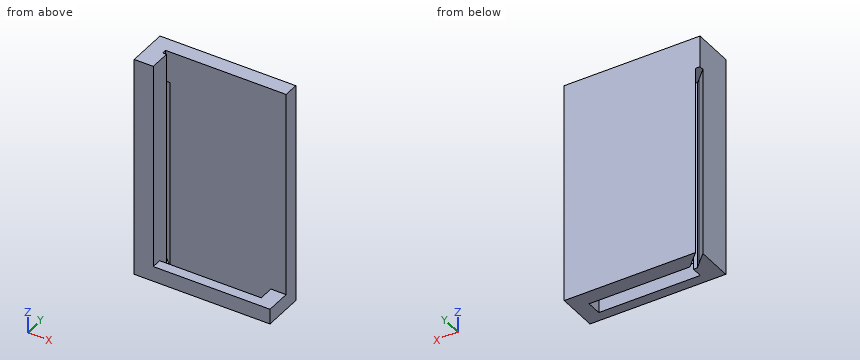
from build123d import *

# Parameters (mm, degrees)
F1_DEPTH = 25
F2_DEPTH = 150
F4_DEPTH = 175
F5_W     = 12
F5_H     = 8
F5_H_2   = 12
F6_DEPTH = 12


with BuildPart() as f1:
    # F0 (on Top) → F1 (new body)
    with BuildSketch(Plane.XY):
        Polygon((-15.4107665035, -11.7272357842), (-11.8752325976, -15.2627696901), (79.5892334965, -15.2627696901), (79.5892334965, -3.2627696901), (-15.4107665035, -3.2627696901), align=None)
        Polygon((-23.8752325976, -3.2627696901), (-15.4107665035, -11.7272357842), (-15.4107665035, -3.2627696901), align=None)
        Polygon((-18.9463004094, -15.2627696901), (-15.4107665035, -15.2627696901), (-27.4107665035, -3.2627696901), (-27.4107665035, -6.7983035961), align=None)
        Polygon((-27.4107665035, -15.2627696901), (-18.9463004094, -15.2627696901), (-27.4107665035, -6.7983035961), align=None)
        Polygon((-15.4107665035, -18.7983035961), (-18.9463004094, -15.2627696901), (-27.4107665035, -15.2627696901), (-27.4107665035, -35.2627696901), (-15.4107665035, -35.2627696901), align=None)
        Polygon((-27.4107665035, -3.2627696901), (-15.4107665035, -15.2627696901), (-15.4107665035, -11.7272357842), (-23.8752325976, -3.2627696901), align=None)
        Polygon((-15.4107665035, -11.7272357842), (-15.4107665035, -15.2627696901), (-11.8752325976, -15.2627696901), align=None)
        Polygon((-15.4107665035, -18.7983035961), (-15.4107665035, -15.2627696901), (-18.9463004094, -15.2627696901), align=None)
    extrude(amount=F1_DEPTH)

    # F0 (on Top) → F2 (join)
    with BuildSketch(Plane.XY):
        Polygon((-15.4107665035, -18.7983035961), (-18.9463004094, -15.2627696901), (-27.4107665035, -15.2627696901), (-27.4107665035, -35.2627696901), (-15.4107665035, -35.2627696901), align=None)
        Polygon((-23.8752325976, -3.2627696901), (-15.4107665035, -11.7272357842), (-15.4107665035, -3.2627696901), align=None)
        Polygon((-15.4107665035, -11.7272357842), (-11.8752325976, -15.2627696901), (79.5892334965, -15.2627696901), (79.5892334965, -3.2627696901), (-15.4107665035, -3.2627696901), align=None)
        Polygon((-27.4107665035, -15.2627696901), (-18.9463004094, -15.2627696901), (-27.4107665035, -6.7983035961), align=None)
    extrude(amount=-F2_DEPTH)

    # F3 (on face) → F4 (join, through all)
    with BuildSketch(Plane(origin=(0, 0, -150), x_dir=(1, 0, 0), z_dir=(0, 0, -1))):
        Polygon((-15.4107665035, 30.7983035961), (-15.4107665035, 18.7983035961), (-12.4107665035, 18.7983035961), (-12.4107665035, 30.7983035961), (-12.4107665035, 35.2627696901), (-15.4107665035, 35.2627696901), align=None)
    extrude(amount=-F4_DEPTH)

    # F5 (on face) → F6 (join)
    with BuildSketch(Plane(origin=(0, 0, -150), x_dir=(1, 0, 0), z_dir=(0, 0, -1))):
        Polygon((-12.4107665035, 35.2627696901), (-12.4107665035, 30.7983035961), (-12.4107665035, 27.2627696901), (67.5892334965, 27.2627696901), (67.5892334965, 35.2627696901), align=None)
        with Locations((73.5892334965, 31.2627696901)):
            Rectangle(F5_W, F5_H)
        with Locations((73.5892334965, 21.2627696901)):
            Rectangle(F5_W, F5_H_2)
        Polygon((79.5892334965, 15.2627696901), (67.5892334965, 15.2627696901), (-11.8752325976, 15.2627696901), (-23.8752325976, 3.2627696901), (79.5892334965, 3.2627696901), align=None)
    extrude(amount=-F6_DEPTH)


solid = f1.part
Geometry: final body of the model. Coordinates: model frame, mm. Round coordinates to 2 decimals unless told otherwise and drop trailing zeros. Loops run counter-clockwise (first coordinate to the right, second up) from the corner with the lowest first, then second, coordinate; pieces in that order, holes last.
Q1. Material intervals for L1, parallel to Z at x = 50, y = -31; L2, parallel to Y at x = 37, z = -90.5; L3, parallel to X at y = -7, z = -120.5, sorted ascending.
Q2. Pin query (flat end, axial travel): P1, Ø3, axis at y = -23, z = 0, coming from the +X side; P2, Ø6, axis at x = -6, y = -21.5, coming from the -Z side; P3, Ø12, axis at x = 68, y = -24.5, coming from the +Z side. Return the tip coordinate at first contact, or that it passes through.
Q3. Section D-D on x = 71.5. Return loops of the section in (y, z), plus the area to 3 significant figures.
Q4. Section B-B on x = 13. Return loops of the section in (y, z).
Q5. Section C-C on y = -23.5. Return loops of the section in (x, z).
Q6. Section A-A on z = -85. Return loops of the section in (x, y), plus the area to 3 significant figures.
Evaluation:
1. L1: z = -150 to -138
1. L2: y = -15.26 to -3.26
1. L3: x = -27.41 to -27.21, -20.14 to 79.59
2. P1: stops at x = -12.41
2. P2: passes through
2. P3: stops at z = -138
3. outline: (-35.26, -150) - (-3.26, -150) - (-3.26, 25) - (-15.26, 25) - (-15.26, -138) - (-35.26, -138) - close
3. area: 2,340 mm2
4. outline: (-35.26, -150) - (-27.26, -150) - (-27.26, -138) - (-35.26, -138) - close; (-15.26, -150) - (-3.26, -150) - (-3.26, 25) - (-15.26, 25) - close
5. outline: (-27.41, -150) - (-12.41, -150) - (-12.41, 25) - (-27.41, 25) - close; (67.59, -150) - (79.59, -150) - (79.59, -138) - (67.59, -138) - close
6. outline: (-27.41, -35.26) - (-12.41, -35.26) - (-12.41, -18.8) - (-15.41, -18.8) - (-27.41, -6.8) - close; (-23.88, -3.26) - (-11.88, -15.26) - (79.59, -15.26) - (79.59, -3.26) - close
6. area: 1,490 mm2
